The model under review builds one solid part; all positions refer to its coordinate system, in mm. A direction names the side the tool comes from. Round coordinates to 2 decimals unless told otherwise and drop trailing zeros. Loops run counter-clockwise (first coordinate to the right, second up) from the corner with the lowest first, then second, coordinate; pieces in that order, holes last. Notation, with made-up numbers: M 41.5,66.25 L 75.5,66.25 A14 cw 75.5,92.25 Z; hole C 29.5,-7 d9. An arc over 180 degrees is marked long. Return JSON: item names as keys, results as strings. Group by question number.
Q1. Clearance check with flat-ended pins moving along their axes: pin 1 Ø6 at (y, z) = (-24, -39) entering from -X; pin 2 Ø10 at (y, z) = (-28, -37.5) entering from +X; pin 3 Ø8 at (x, y) = (9.5, -30) entering from +Z; pin 4 Ø1 at (x, y) = (-8, -18.5) entering from -Z. State where each tip first meets the part, or that it passes through.
Q2. Consider section C-C (z = -39.5). State the section outline as (x, y) points, and give its area (3 significant figures).
Q3. Consider section D-D (x = 15.5). State the section outline as (y, z) points, and give its area (3 significant figures).
Q4. Consider section A-A (y = -34). State the section outline as (x, z) points, and give its area (3 significant figures).
Q5. Draft analysis for pull direction X (two halves, no side actions). For faces 1 (the face through (-13.25, -27, -48)), 2 (the face through (22.5, -10, -28)), 3 (the face through (-14.77, -21.26, -40.49)), state which applies: pulls with the +X half, pulls with the -X half, needs draft (parallel to the pull), parting line crosses it, or undercut.
Q6. For faces 4 (the face through (15, -27, -26)), 5 (the face through (16.25, -27, -48)), 6 (the face through (0, -9, -58)), 7 (the face through (13.25, -27, -48)), list the 3-axis set-ups (+Z, -Z, +X, -X, +Y, -Y) from which the entire face can be reached by the end or side of a thin tool; tool diameter is ignored.
Q7. Consider section B-B (y = -26.5). State the section outline as (x, z) points.
Q8. To check wall thickness, follow line 1 along X through (y, z) = (-29, -55); line 2 along Y through (x, z) = (-15.4, -59.8); line 3 along Y through (x, z) = (16, -13). State the ranges of each line that lie inside material, in increasing order.
from build123d import *

# Parameters (mm, degrees)
BOSS_EXTRUDE1_DEPTH = 22.5
SKETCH2_W           = 3
SKETCH2_H           = 44
BOSS_EXTRUDE2_DEPTH = 20.5
SKETCH3_R           = 1.25
CUT_EXTRUDE1_DEPTH  = 39.75


with BuildPart() as part:
    # Sketch1 → Boss-Extrude1 (new body, symmetric)
    with BuildSketch(Plane(origin=(0, 0, 0), x_dir=(0, 0, -1), z_dir=(1, 0, 0))):
        with BuildLine():
            Line((5, 0), (30, 0))
            Line((30, 0), (45.588457268, -9))
            Line((45.588457268, -9), (70, -9))
            Line((70, -9), (70, -17))
            Line((70, -17), (63.318457268, -17))
            Line((63.318457268, -17), (0, -17))
            Line((0, -17), (0, -5))
            ThreePointArc((0, -5), (1.464466094, -1.464466094), (5, 0))
        make_face()
    extrude(amount=BOSS_EXTRUDE1_DEPTH, both=True)

    # Sketch2 → Boss-Extrude2 (add)
    with BuildSketch(Plane.XZ.offset(17)):
        with Locations((14.75, -48)):
            Rectangle(SKETCH2_W, SKETCH2_H)
        with Locations((-14.75, -48)):
            Rectangle(SKETCH2_W, SKETCH2_H)
    extrude(amount=BOSS_EXTRUDE2_DEPTH)

    # Sketch3 → Cut-Extrude1 (cut, through all)
    with BuildSketch(Plane.ZY.offset(16.25)):
        with Locations((-59.8, -34)):
            Circle(SKETCH3_R)
        with Locations((-39.5, -20.5)):
            Circle(SKETCH3_R)
    extrude(amount=-CUT_EXTRUDE1_DEPTH, mode=Mode.SUBTRACT)


solid = part.part
Values:
{
 "1": {"pin 1": "stops at x = -16.25", "pin 2": "stops at x = 16.25", "pin 3": "stops at z = -26", "pin 4": "passes through"},
 "2": {"outline": "M -22.5,-17 L -16.25,-17 L -16.25,-19.25 L -13.25,-19.25 L -13.25,-17 L 13.25,-17 L 13.25,-19.25 L 16.25,-19.25 L 16.25,-17 L 22.5,-17 L 22.5,-5.48 L -22.5,-5.48 Z; M -16.25,-37.5 L -13.25,-37.5 L -13.25,-21.75 L -16.25,-21.75 Z; M 13.25,-37.5 L 16.25,-37.5 L 16.25,-21.75 L 13.25,-21.75 Z", "area": "626 mm2"},
 "3": {"outline": "M -37.5,-70 L -9,-70 L -9,-45.59 L 0,-30 L 0,-5 A5 ccw -5,0 L -17,0 L -17,-26 L -37.5,-26 Z; hole C -34,-59.8 d2.5; hole C -20.5,-39.5 d2.5", "area": "1,790 mm2"},
 "4": {"outline": "M -16.25,-70 L -13.25,-70 L -13.25,-61.05 L -16.25,-61.05 Z; M -16.25,-58.55 L -13.25,-58.55 L -13.25,-26 L -16.25,-26 Z; M 13.25,-70 L 16.25,-70 L 16.25,-61.05 L 13.25,-61.05 Z; M 13.25,-58.55 L 16.25,-58.55 L 16.25,-26 L 13.25,-26 Z", "area": "249 mm2"},
 "5": {"face 1": "undercut", "face 2": "pulls with the +X half", "face 3": "needs draft"},
 "6": {"face 4": "+Z, +X, -X, -Y", "face 5": "+Z, -Z, +X, -Y", "face 6": "-Z, +X, -X, +Y", "face 7": "+Z, -Z, -Y"},
 "7": {"outline": "M -16.25,-70 L -13.25,-70 L -13.25,-26 L -16.25,-26 Z; M 13.25,-70 L 16.25,-70 L 16.25,-26 L 13.25,-26 Z"},
 "8": {"line 1": "x = -16.25 to -13.25, 13.25 to 16.25", "line 2": "y = -37.5 to -35.25, -32.75 to -9", "line 3": "y = -17 to 0"}
}
